Autodesk Inventor part; units mm, degrees
ref_plane "Work Plane1" through (13.32, 0, 0) normal (0, 0, 1) x (-1, 0, 0)
ref_plane "YZ Plane" through (0, 0, 0) normal (1, 0, 0) x (0, 1, 0)
ref_plane "XZ Plane" through (0, 0, 0) normal (0, 1, 0) x (-1, 0, 0)
sketch "Sketch1" plane through (0, 0, 0) normal (1, 0, 0) x (0, 1, 0)
  line L0 (-4.6188, 0) -> (-2.3094, 4)
  line L1 (-2.3094, 4) -> (2.3094, 4)
  line L2 (2.3094, 4) -> (4.6188, 0)
  line L3 (4.6188, 0) -> (2.3094, -4)
  line L4 (2.3094, -4) -> (-2.3094, -4)
  line L5 (-2.3094, -4) -> (-4.6188, 0)
  point P0 (0, 0)
  point P1 (0, 0)
  dimension "d0" = 9.2376
extrude "Body" add sketch "Sketch1" along normal blind 5.3
sketch "Sketch2" plane through (0, 0, 0) normal (-1, 0, 0) x (0, 0, 1)
  line L0 (0, -6.4663) -> (0, 6.4663)
  line L1 (-5.6, 0) -> (5.6, 0)
  point P0 (0, 0)
hole "Thread" at (0, 0, 0) direction (1, 0, 0) diameter 4.134 end through all
chamfer "Chamfer1" distance 0.433 angle 30 1 edges at (0, 0, -2.067) measured on face at (0, -2.8764, -1.7247)
chamfer "Chamfer2" distance 0.433 angle 30 1 edges at (5.3, 0, -2.067) measured on face at (5.3, -2.8764, -1.7247)
sketch "Sketch3" plane through (0, 0, 0) normal (0, 0, 1) x (1, 0, 0)
  line L0 (0, 2.3094) -> (0, 4.6188)
  line L1 (0, 4.6188) -> (5.3, 4.6188)
  line L2 (5.3, 2.3094) -> (5.3, 4.6188)
  line L3 (-1.06, 0) -> (6.36, 0)
  line L4 (0.3573, 4.6188) -> (0, 4)
  line L5 (5.3, 3.4) -> (4.1525, 3.4)
  line L6 (4.1525, 3.4) -> (2.7, 4.6188)
  dimension "d3" = 30
  dimension "d5" = 8
  dimension "d6" = 6.8
  dimension "d8" = 50
  dimension "d9" = 2.7
revolve "Chamfer3" cut sketch "Sketch3" angle 360 about axis through (-10, 0, 0) along (1, 0, 0)
ref_plane "Work Plane1" through (13.32, 0, 0) normal (0, 0, 1) x (-1, 0, 0)
equation "\"d0\" = 1.1547 * SW"
equation "\"d1\" = KOH"
equation "\"d3\" = ANG1"
equation "\"d5\" = SW0"
equation "\"d6\" = SW1"
equation "\"d8\" = ANG2"
equation "\"d9\" = KOH1"
equation "\"d10\" = -0.5 * GD1 + 0.5 * NND"
equation "\"d39\" = -0.5 * GD1 + 0.5 * NND"
equation "\"d12\" = -0.5 * GD1 + 0.5 * NND"
equation "\"d40\" = -0.5 * GD1 + 0.5 * NND"
equation "\"ANG1\" = 30deg"
equation "\"ANG2\" = 50deg"
equation "\"NND\" = 5"
equation "\"KOH\" = 5.3"
equation "\"SW\" = 8"
equation "\"SW0\" = SW"
equation "\"SW1\" = 0.85 * SW"
equation "\"KOH1\" = 2.7"
equation "\"GUL\" = 0.541266 * PTC"
equation "\"THREADDIA\" = 5"
equation "\"TOA\" = 30deg"
equation "\"PTC\" = 0.8"
equation "\"E0\" = 1.155 * SW"
equation "\"GAL\" = 0.541266 * PTC"
properties part number "ANSI B18.16.3M - Property Class 9 - Metric M5 x 0.8 Metal Type" material "Steel, Mild"
Read the model definition and answer for the solid it produces. Units are mm, in the model's axes. Round coordinates to 2 decimals unless told otherwise and drop trailing zeros. Order: outer loops, then holes, each group sorted by start corner. A loop starts at its lowest first (then second) coordinate and runs counter-clockwise, first axis right, second up.
1) The part is cut by section B-B on x = 4.9. Write down the section's boundary in (y, z), plus the area to 3 significant figures.
2) The part is cut by section A-A on x = 2.45. Write down the section's boundary in (y, z).
3) Flat-ended cylindrical pins translate along their axes: pin 1 (2 mm diameter, centred on x = 3.5, z = 2, fed in from -Y); pin 2 (1 mm diameter, centred on x = 3.5, z = -0.5, fed in from +Y). Find the tip coordinate at first contact, or state that the pin passes through.
4) Straight lines are drawn through the part: L1, parallel to Z at x = 1.6, y = 0; L2, parallel to Y at x = 3.35, z = 0; L3, parallel to Y at x = 3.9, z = 0. For each, find the intervals that lie inside material, in ascending order.
5) The mould has two halves that part along Y. Classify faces 1 (the face through (0.087, 4.15, -0.01)), 2 (the face through (4.72, -0.74, 3.32)), 3 (the face through (2.68, 1.26, -1.64)): released by +Y, released by -Y, zero draft, split by the parting line, or undercut.
Resolved:
1. outline: circle Ø6.8 at (0, 0); hole circle Ø4.13 at (0, 0)
1. area: 22.9 mm2
2. outline: (-4.62, 0) - (-2.31, -4) - (2.31, -4) - (4.62, 0) - (2.31, 4) - (-2.31, 4) - close; hole circle Ø4.13 at (0, 0)
3. pin 1: stops at y = -4.02
3. pin 2: stops at y = 4.34
4. L1: z = -4 to -2.07, 2.07 to 4
4. L2: y = -4.07 to -2.07, 2.07 to 4.07
4. L3: y = -3.61 to -2.07, 2.07 to 3.61
5. face 1: released by +Y
5. face 2: split by the parting line
5. face 3: undercut
